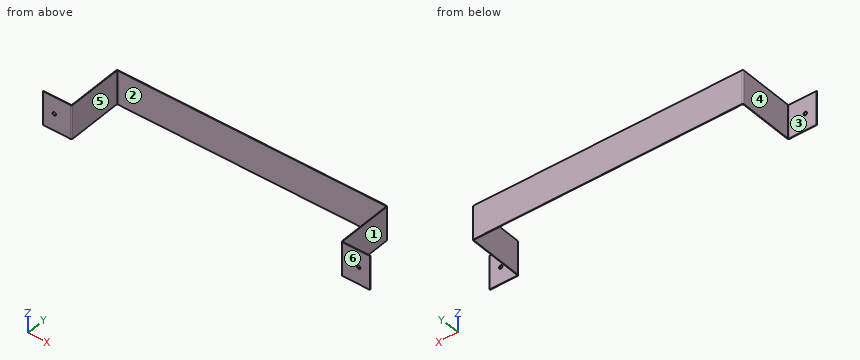
```python
from build123d import *

# Parameters (mm, degrees)
BASE_FLANGE1_DEPTH = 30
SKETCH6_R          = 1.5
CUT_EXTRUDE1_DEPTH = 10


# Sheet-metal steps are written as plain solids
with BuildPart() as part:
    # Sketch1 → Base-Flange1 (new body)
    with BuildSketch(Plane.XY):
        with BuildLine():
            Line((-145, 0), (-120.5, 0))
            ThreePointArc((-120.5, 0), (-120.146446609, 0.146446609), (-120, 0.5))
            Line((-120, 0.5), (-120, 49))
            ThreePointArc((-120, 49), (-119.707106781, 49.707106781), (-119, 50))
            Line((-119, 50), (119, 50))
            ThreePointArc((119, 50), (119.707106781, 49.707106781), (120, 49))
            Line((120, 49), (120, 0.5))
            ThreePointArc((120, 0.5), (120.146446609, 0.146446609), (120.5, 0))
            Line((120.5, 0), (145, 0))
            Line((145, 0), (145, -0.5))
            Line((145, -0.5), (120.5, -0.5))
            ThreePointArc((120.5, -0.5), (119.792893219, -0.207106781), (119.5, 0.5))
            Line((119.5, 0.5), (119.5, 49))
            ThreePointArc((119.5, 49), (119.353553391, 49.353553391), (119, 49.5))
            Line((119, 49.5), (-119, 49.5))
            ThreePointArc((-119, 49.5), (-119.353553391, 49.353553391), (-119.5, 49))
            Line((-119.5, 49), (-119.5, 0.5))
            ThreePointArc((-119.5, 0.5), (-119.792893219, -0.207106781), (-120.5, -0.5))
            Line((-120.5, -0.5), (-145, -0.5))
            Line((-145, -0.5), (-145, 0))
        make_face()
    extrude(amount=BASE_FLANGE1_DEPTH)

    # Sketch6 → Cut-Extrude1 (cut)
    with BuildSketch(Plane(origin=(0, 0, 0), x_dir=(1, 0, 0), z_dir=(0, 1, 0))):
        with Locations(Location((135, -15, 0), (0, 0, 270))):
            Circle(SKETCH6_R)
        with Locations(Location((-135, -15, 0), (0, 0, 90))):
            Circle(SKETCH6_R)
    extrude(amount=-CUT_EXTRUDE1_DEPTH, mode=Mode.SUBTRACT)


solid = part.part
```
Part model, mm, in its own coordinate system. Face numbers are marked on the shaded views. A direction names the side the tool comes from. Round coordinates to 2 decimals unless told otherwise and drop trailing zeros. Write each loop counter-clockwise with the first axis right and the second up, starting at its lowest first coordinate (ties: lowest second). Pieces come first, ordered by that corner, then holes. Notation, with made-up numbers: (79, 75.5) -> (105, 75.5) arc R30 ccw to (105, 105.5) -> close; hole circle Ø6 at (31, 52.5). An arc over 180 degrees is marked (long way). Return JSON: item names as keys, results as strings. Group by question number.
Q1. Mould opens along X. For the marked faces 4, 5 and 6 say: pulls with the +X half, pulls with the -X half, needs draft (parallel to the pull), parting line crosses it, or undercut.
Q2. Probe L1, parallel to Z at x = 135, y = -0.1; L2, parallel to X at y = 3, z = 6; L3, parallel to X at y = -0.2, z = 15. List the from-to ranges inside material, lowest first. Write a range as [from, to].
Q3. Pin check, flat tips, straight feed: pin 1 (15 mm diameter, centred on x = 9.5, z = 12.5, fed in from -Y); pin 2 (9 mm diameter, centred on y = 26, z = 16.5, fed in from +X); pin 3 (12 mm diameter, centred on x = 133.5, z = 22.5, fed in from +Y); pin 4 (4 mm diameter, centred on x = -135, z = 15, fed in from -Y). Stop position of each tip, or through.
Q4. Saw through at A-A on y = 26.5. Write the cut outline in (x, z).
Q5. Saw through at B-B on z = 20.25. Write the cut outline in (x, y), plus the area to 3 significant figures.
Q6. Which spindle directions (+Z, -Z, +X, -X, +Y, -Y) get a long thin tool onto all of the face, cutting with end or side? Do the marked faces 1, 2 and 3. Say none if no direction does.
Q7. Saw through at C-C on x = 57.5. Write the cut outline in (y, z).
Answer:
{
 "1": {"face 4": "pulls with the -X half", "face 5": "undercut", "face 6": "needs draft"},
 "2": {"L1": "[0, 13.5], [16.5, 30]", "L2": "[-120, -119.5], [119.5, 120]", "L3": "[-145, -136.5], [-133.5, -119.79], [119.79, 133.5], [136.5, 145]"},
 "3": {"pin 1": "y = 49.5", "pin 2": "x = 120", "pin 3": "y = 0", "pin 4": "y = -0.5"},
 "4": {"outline": "(-120, 0) -> (-119.5, 0) -> (-119.5, 30) -> (-120, 30) -> close; (119.5, 0) -> (120, 0) -> (120, 30) -> (119.5, 30) -> close"},
 "5": {"outline": "(-145, -0.5) -> (-120.5, -0.5) arc R1 ccw to (-119.5, 0.5) -> (-119.5, 49) arc R0.5 cw to (-119, 49.5) -> (119, 49.5) arc R0.5 cw to (119.5, 49) -> (119.5, 0.5) arc R1 ccw to (120.5, -0.5) -> (145, -0.5) -> (145, 0) -> (120.5, 0) arc R0.5 cw to (120, 0.5) -> (120, 49) arc R1 ccw to (119, 50) -> (-119, 50) arc R1 ccw to (-120, 49) -> (-120, 0.5) arc R0.5 cw to (-120.5, 0) -> (-145, 0) -> close", "area": "194 mm2"},
 "6": {"face 1": "+Z, -Z, +X, +Y", "face 2": "+Z, -Z, -Y", "face 3": "+Z, -Z, -X, +Y"},
 "7": {"outline": "(49.5, 0) -> (50, 0) -> (50, 30) -> (49.5, 30) -> close"}
}
